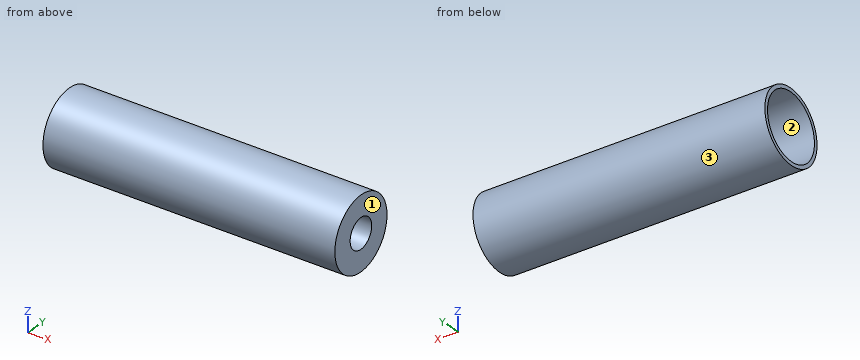
Autodesk Inventor part; units mm, degrees
ref_plane "YZ Plane" through (0, 0, 0) normal (1, 0, 0) x (0, 1, 0)
ref_plane "XZ Plane" through (0, 0, 0) normal (0, 1, 0) x (-1, 0, 0)
ref_plane "XY Plane" through (0, 0, 0) normal (0, 0, 1) x (1, 0, 0)
sketch "Sketch1" plane through (0, 0, 0) normal (1, 0, 0) x (0, 1, 0)
  circle A0 centre (0, 0) radius 5
  dimension "d0" = 10
extrude "Extrusion1" add sketch "Sketch1" along normal blind 40
sketch "Sketch2" plane through (40, 0, 0) normal (1, 0, 0) x (0, 0, -1)
  point P0 (0, 0)
  point P1 (0, 0)
hole "Hole1" at (40, 0, 0) direction (-1, 0, 0) diameter 4.134 depth 10 tip angle 118
sketch "Sketch3" plane through (0, 0, 0) normal (-1, 0, 0) x (0, 0, 1)
  point P0 (0, 0)
  point P1 (0, 0)
hole "Hole2" at (0, 0, 0) direction (1, 0, 0) diameter 9 depth 25 tip angle 118
properties part number "CopleCatheter"
Geometry check sheet. Reference: the model listing, model coordinates, mm. Face numbers are marked on the shaded views. Give positions to 0.01 mm unless a question says otherwise; leave off trailing zeros. Order: outer loops, then holes, each group sorted by start corner. A loop starts at its lowest first (then second) coordinate and runs counter-clockwise, first axis right, second up. Notation, with made-up numbers: (56.5, 82) - (88.5, 82) arc R19 ccw to (88.5, 117) - close; hole circle Ø6 at (65.5, -23). An arc over 180 degrees is marked (long way). Answer as a JSON object with one key per item and string values.
(1) Material ranges on line 1 (Z direction, x = 33.75, y = 0); line 2 (Z direction, x = 18, y = 0); line 3 (Y direction, x = 5.5, z = 1.25), recorded low to high.
Report:
{"line 1": "-5 to -2.07, 2.07 to 5", "line 2": "-5 to -4.5, 4.5 to 5", "line 3": "-4.84 to -4.32, 4.32 to 4.84"}
(2) Depth check by flat-ended pin: pin 1 Ø1 at (x, z) = (21, 3) entering from +Y; pin 2 Ø4 at (x, y) = (16, 1.5) entering from +Z; pin 3 Ø2 at (x, z) = (27.5, 3) entering from -Y; pin 4 Ø3.5 at (y, z) = (0, 0) entering from -X. Enter the tip coordinate at first touch or a pass-through.
Report:
{"pin 1": "y = 4.33", "pin 2": "z = 5", "pin 3": "y = -4.58", "pin 4": "x = 26.65"}
(3) Cross-section at A-A (x = 8.5). Record the cut outline in (y, z), then the cut area to 3 significant figures.
Report:
{"outline": "circle Ø10 at (0, 0); hole circle Ø9 at (0, 0)", "area": "14.9 mm^2"}
(4) Draft check along Y on the marked faces 1, 2 and 3. Enter one of: released by +Y, released by -Y, zero draft, split by the parting line, or undercut.
Report:
{"face 1": "zero draft", "face 2": "undercut", "face 3": "split by the parting line"}
